from build123d import *

# Parameters (mm, degrees)
F1_DEPTH  = 2.5
F2_W      = 30.8
F2_H      = 24.25
F3_DEPTH  = 1.5
F4_DEPTH  = 1.5
F5_W      = 1
F5_H      = 2
F6_DEPTH  = 28.251
F7_W      = 1
F7_H      = 2
F8_DEPTH  = 28.251
F9_W      = 1
F9_H      = 2
F10_DEPTH = 33.801
F11_W     = 1
F11_H     = 2
F12_DEPTH = 33.801
F15_R     = 1
F13_R     = 1
F16_R     = 1
F17_DEPTH = 8.1
F18_W     = 34.8
F18_H     = 28.25
F18_W_2   = 34.6
F18_H_2   = 28.05
F19_DEPTH = 1
F20_R     = 2
F21_DEPTH = 4.001


with BuildPart() as f1:
    # F0 (on Top) → F1 (new body)
    with BuildSketch(Plane.XY):
        Polygon((-17.4, 14.125), (-17.4, -14.125), (0, 0), align=None)
        Polygon((0, 0), (-17.4, -14.125), (17.4, -14.125), align=None)
        Polygon((0, 0), (17.4, -14.125), (17.4, 14.125), align=None)
        Polygon((17.4, 14.125), (-17.4, 14.125), (0, 0), align=None)
    extrude(amount=F1_DEPTH)

    # F2 (on face) → F3 (cut)
    with BuildSketch(Plane.XY.offset(2.5)):
        Rectangle(F2_W, F2_H)
    extrude(amount=-F3_DEPTH, mode=Mode.SUBTRACT)

    # F4 (add): a face of the model
    f4_faces = [f1.faces().sort_by_distance(p)[0] for p in [
        (-16.9517698694, 0, 2.5),
    ]]
    extrude(f4_faces, amount=F4_DEPTH)

    # F5 (on face) → F6 (cut, through all)
    with BuildSketch(Plane.XZ.offset(14.125)):
        with Locations((-16.9, 2)):
            Rectangle(F5_W, F5_H)
    extrude(amount=-F6_DEPTH, mode=Mode.SUBTRACT)

    # F7 (on face) → F8 (cut, through all)
    with BuildSketch(Plane.XZ.offset(14.125)):
        with Locations((16.9, 2)):
            Rectangle(F7_W, F7_H)
    extrude(amount=-F8_DEPTH, mode=Mode.SUBTRACT)

    # F9 (on face) → F10 (cut, through all)
    with BuildSketch(Plane(origin=(-16.4, 0, 0), x_dir=(0, -1, 0), z_dir=(-1, 0, 0))):
        with Locations((13.625, 2)):
            Rectangle(F9_W, F9_H)
    extrude(amount=-F10_DEPTH, mode=Mode.SUBTRACT)

    # F11 (on face) → F12 (cut, through all)
    with BuildSketch(Plane.YZ.offset(16.4)):
        with Locations((13.625, 2)):
            Rectangle(F11_W, F11_H)
    extrude(amount=-F12_DEPTH, mode=Mode.SUBTRACT)

    # F15 (on face) + F13 (on face) + F16 (on face) → F17 (join)
    with BuildSketch(Plane(origin=(0, 0, 0), x_dir=(1, 0, 0), z_dir=(0, 0, -1))):
        with Locations((-13.4, -10.125)):
            Circle(F15_R)
        with Locations((-13.4, 10.125)):
            Circle(F15_R)
    with BuildSketch(Plane(origin=(0, 0, 0), x_dir=(1, 0, 0), z_dir=(0, 0, -1))):
        with Locations((13.4, -10.125)):
            Circle(F13_R)
    with BuildSketch(Plane(origin=(0, 0, 0), x_dir=(1, 0, 0), z_dir=(0, 0, -1))):
        with Locations((13.4, 10.125)):
            Circle(F16_R)
    extrude(amount=F17_DEPTH)

    # F18 (on face) → F19 (cut, through all)
    with BuildSketch(Plane(origin=(0, 0, 0), x_dir=(1, 0, 0), z_dir=(0, 0, -1))):
        Rectangle(F18_W, F18_H)
        Rectangle(F18_W_2, F18_H_2, mode=Mode.SUBTRACT)
    extrude(amount=-F19_DEPTH, mode=Mode.SUBTRACT)

    # F20 (on face) → F21 (cut, through all)
    with BuildSketch(Plane(origin=(0, 0, 0), x_dir=(1, 0, 0), z_dir=(0, 0, -1))):
        with Locations((9.3, -6.025)):
            Circle(F20_R)
    extrude(amount=-F21_DEPTH, mode=Mode.SUBTRACT)


solid = f1.part
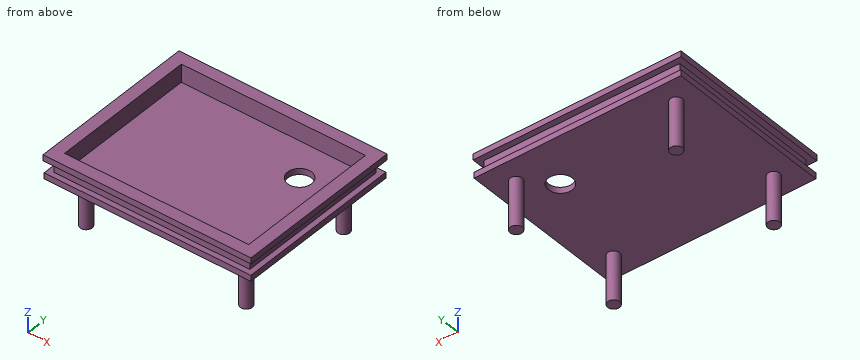
Source: CAD feature listing. Evaluate the final solid. Frame: model axes, mm. Give positions to 0.01 mm unless a question says otherwise; leave off trailing zeros. Write each loop counter-clockwise with the first axis right and the second up, starting at its lowest first coordinate (ties: lowest second). Pieces come first, ordered by that corner, then holes. Notation, with made-up numbers: M -6.75,49.5 L 19.25,49.5 A26 ccw 19.25,79.5 Z; hole C 10,17.5 d2. An arc over 180 degrees is marked long. Answer as a JSON object with one key per item and string values.
Q1. Cut plane D-D, the plane x = 1. Return the cut outline in (y, z) (3 decimals).
Geometry check:
{"outline": "M -14.125,3 L -13.125,3 L -13.125,1 L -14.025,1 L -14.025,0 L 14.025,0 L 14.025,1 L 13.125,1 L 13.125,3 L 14.125,3 L 14.125,4 L 12.125,4 L 12.125,1 L -12.125,1 L -12.125,4 L -14.125,4 Z"}
Q2. Contact query for flat-ended pins moving along their axis: P1, Ø0.5, axis at x = -3.5, z = 0.5, coming from the -Y side (3 decimals); P2, Ø1, axis at x = -5.5, y = 6, coming from the +Z side; P3, Ø0.6, axis at y = -3, z = 2.5, coming from the +X side. Output: stop coordinate, or through.
Geometry check:
{"P1": "stops at y = -14.025", "P2": "stops at z = 1", "P3": "stops at x = 16.4"}
Q3. Cut plane B-B, the plane x = 9.3. Return the cut outline in (y, z) (3 decimals), then the cut area to 4 significant figures.
Geometry check:
{"outline": "M -14.125,3 L -13.125,3 L -13.125,1 L -14.025,1 L -14.025,0 L 4.025,0 L 4.025,1 L -12.125,1 L -12.125,4 L -14.125,4 Z; M 8.025,0 L 14.025,0 L 14.025,1 L 13.125,1 L 13.125,3 L 14.125,3 L 14.125,4 L 12.125,4 L 12.125,1 L 8.025,1 Z", "area": "32.05 mm^2"}
Q4. Cut plane A-A, the plane z = 2.5. Return the cut outline in (x, y) (3 decimals).
Geometry check:
{"outline": "M -16.4,-13.125 L 16.4,-13.125 L 16.4,13.125 L -16.4,13.125 Z; hole M -15.4,-12.125 L 15.4,-12.125 L 15.4,12.125 L -15.4,12.125 Z"}
Q5. Ray query, line 1 along Y through (x, z) = (11.5, 1.25) (3 decimals); line 2 along X through (y, z) = (-3.75, 1.25); line 3 along X through (y, z) = (-0.25, 0.5). Return the intervals inside material, ascending.
Geometry check:
{"line 1": "y = -13.125 to -12.125, 12.125 to 13.125", "line 2": "x = -16.4 to -15.4, 15.4 to 16.4", "line 3": "x = -17.3 to 17.3"}
Q6. Cut plane C-C, the plane y = -3.5. Return the cut outline in (x, z).
Geometry check:
{"outline": "M -17.4,3 L -16.4,3 L -16.4,1 L -17.3,1 L -17.3,0 L 17.3,0 L 17.3,1 L 16.4,1 L 16.4,3 L 17.4,3 L 17.4,4 L 15.4,4 L 15.4,1 L -15.4,1 L -15.4,4 L -17.4,4 Z"}
